Part model, mm, in its own coordinate system. A direction names the side the tool comes from. Give positions to 0.01 mm unless a question says otherwise; leave off trailing zeros. Write each loop counter-clockwise with the first axis right and the second up, starting at its lowest first coordinate (ties: lowest second). Pieces come first, ordered by that corner, then holes. Notation, with made-up numbers: (42.25, 47.25) - (62.25, 47.25) arc R21 cw to (62.25, 53.25) - close; hole circle Ø6 at (-33, 40). An arc over 180 degrees is marked (long way). Answer in a Markdown table with one row per item. Add a question column.
1. Probe line 1 along Y through (x, z) = (46, 40); line 2 along X through (y, z) = (-23, 30). List the from-to ranges inside material, lowest first.
2. Band-saw the part on C-C on y = -28. Write the cut outline in (x, z), plus the area to 3 significant figures.
3. Which spindle directions (+Z, -Z, +X, -X, +Y, -Y) get a long thin tool onto all of the face, cutting with end or side? Do faces 1 (the cylindrical face through (52.472, 48.551, 40.56)), 2 (the flat face through (50, -1, 39)). Say none if no direction does.
4. Band-saw the part on B-B on z = 41.5. Write the cut outline in (x, y).
5. Pull direction X, two halves, no side cores. Call faces 3 (the flat face through (-4, -48, 80)), 4 (the flat face through (-50, -1, 39)), 5 (the flat face through (54, -1, 39)): released by +X, released by -X, zero draft, split by the parting line, or undercut.
6. Band-saw the part on A-A on x = -4. Write the cut outline in (y, z), plus the area to 3 significant figures.
```python
from build123d import *

# Parameters (mm, degrees)
F0_W     = 108
F0_H     = 100
F0_W_2   = 100
F0_H_2   = 92
F1_DEPTH = 80
F2_R     = 5.08
F3_R     = 5.08


with BuildPart() as f1:
    # F0 (on Top) → F1 (new body)
    with BuildSketch(Plane.XY):
        Rectangle(F0_W, F0_H)
        Rectangle(F0_W_2, F0_H_2, mode=Mode.SUBTRACT)
    extrude(amount=F1_DEPTH)

    # F2
    f2_edges = [f1.edges().sort_by_distance(p)[0] for p in [
        (-54, -50, 40),
    ]]
    fillet(f2_edges, radius=F2_R)

    # F3
    f3_edges = [f1.edges().sort_by_distance(p)[0] for p in [
        (54, -50, 40),
        (54, 50, 40),
        (-54, 50, 40),
    ]]
    fillet(f3_edges, radius=F3_R)


solid = f1.part
```
Values:
| question | item | result |
|---|---|---|
| 1 | line 1 | y = -50 to -46, 46 to 50 |
| 1 | line 2 | x = -54 to -50, 50 to 54 |
| 2 | outline | (-54, 0) - (-50, 0) - (-50, 80) - (-54, 80) - close; (50, 0) - (54, 0) - (54, 80) - (50, 80) - close |
| 2 | area | 640 mm² |
| 3 | face 1 | +Z, -Z, +X, +Y |
| 3 | face 2 | +Z, -Z |
| 4 | outline | (-54, -44.92) arc R5.08 ccw to (-48.92, -50) - (48.92, -50) arc R5.08 ccw to (54, -44.92) - (54, 44.92) arc R5.08 ccw to (48.92, 50) - (-48.92, 50) arc R5.08 ccw to (-54, 44.92) - close; hole (-50, -46) - (50, -46) - (50, 46) - (-50, 46) - close |
| 5 | face 3 | zero draft |
| 5 | face 4 | undercut |
| 5 | face 5 | released by +X |
| 6 | outline | (-50, 0) - (-46, 0) - (-46, 80) - (-50, 80) - close; (46, 0) - (50, 0) - (50, 80) - (46, 80) - close |
| 6 | area | 640 mm² |
